from build123d import *

# Parameters (mm, degrees)
BOSS_EXTRUDE1_DEPTH = 15
CUT_EXTRUDE2_DEPTH  = 10
FILLET2_R           = 2


with BuildPart() as part:
    # Sketch1 → Boss-Extrude1 (new body)
    with BuildSketch(Plane(origin=(0, 0, 0), x_dir=(1, 0, 0), z_dir=(0, 1, 0))):
        Polygon((-2, 0), (-2, 30), (-11, 30), (-11, 35), (2, 35), (2, 30), (2, 0), (-4.698729811, -25), (-8.698729811, -25), (-3.876557728, -7.003408785), (-18.977490779, -25), (-22.977490779, -25), align=None)
    extrude(amount=BOSS_EXTRUDE1_DEPTH)

    # Sketch3 → Cut-Extrude2 (cut)
    with BuildSketch(Plane(origin=(0, 0, -35), x_dir=(-1, 0, 0), z_dir=(0, 0, -1))):
        with BuildLine():
            ThreePointArc((8.85, 7.5), (8.611041293, 8.341169779), (7.965541753, 8.931083506))
            Line((7.965541753, 8.931083506), (6.534458247, 6.068916494))
            ThreePointArc((6.534458247, 6.068916494), (8.091169779, 6.138958707), (8.85, 7.5))
        make_face()
        with BuildLine():
            Line((6.534458247, 6.068916494), (7.965541753, 8.931083506))
            ThreePointArc((7.965541753, 8.931083506), (5.818916494, 8.215541753), (6.534458247, 6.068916494))
        make_face()
    extrude(amount=-CUT_EXTRUDE2_DEPTH, mode=Mode.SUBTRACT)

    # Fillet2
    fillet2_edges = [part.edges().sort_by_distance(p)[0] for p in [
        (-2, 7.5, 0),
        (-2, 7.5, -30),
        (2, 7.5, 0),
        (-3.876557728, 7.5, 7.003408785),
    ]]
    fillet(fillet2_edges, radius=FILLET2_R)


solid = part.part
For this review, take the finished solid that the model builds, in its own axes (mm). A direction names the side the tool comes from. Round coordinates to 2 decimals unless told otherwise and drop trailing zeros. Loops run counter-clockwise (first coordinate to the right, second up) from the corner with the lowest first, then second, coordinate; pieces in that order, holes last. Notation, with made-up numbers: (-11.75, 25) - (34.25, 25) arc R26 ccw to (34.25, 62) - close; hole circle Ø9 at (6.25, -27). An arc over 180 degrees is marked (long way). Use one line per item in the form item = value.
1) We need section A-A on x = -7.25. Write out the cut boundary in (y, z).
Solutions:
outline = (0, -35) - (5.9, -35) - (5.9, -30) - (0, -30) - close; (0, 6.26) - (15, 6.26) - (15, 13.41) - (0, 13.41) - close; (0, 19.59) - (15, 19.59) - (15, 25) - (0, 25) - close; (9.1, -35) - (15, -35) - (15, -30) - (9.1, -30) - close
2) Tool access review of faces 5 (the face through (-14.26, 7.4, 19.38)), 6 (the face through (-7.47, 7.4, 20.42)), 7 (the face through (-1, 15, -3)), 8 (the face through (-9, 7, -30)): name each direction out of +Z, -Z, +X, -X, +Y, -Y from which nothing blocks a thin tool from reaching the whole face with its end or side.
Solutions:
face_5 = +Z, +Y, -Y
face_6 = +Y, -Y
face_7 = +Z, -Z, +X, -X, +Y
face_8 = -X, +Y, -Y
3) We need section D-D on z = -5.5. Write out the cut boundary in (x, y).
Solutions:
outline = (-2, 0) - (2, 0) - (2, 15) - (-2, 15) - close
4) Clearance check with flat-ended pins moving along their axes: P1, Ø1.5, axis at x = -2.5, z = -26.5, coming from the +Y side; P2, Ø2, axis at y = 11.5, z = 1.5, coming from the -X side; P3, Ø4, axis at y = 10, z = -31.5, coming from the -X side. State where each tip first meets the part, or that it passes through.
Solutions:
P1 = 15
P2 = -4.1
P3 = -11
5) Wall thickness on probe 1 along X at (y, z) = (11, -20); probe 2 along Z at (x, y) = (-9.75, 3.5); probe 3 along X at (y, z) = (9.75, 23): over which ranges is each line inside the solid? List them lowest first.
Solutions:
probe_1 = -2 to 2
probe_2 = -35 to -30, 9.24 to 14
probe_3 = -21.3 to -17.3, -8.16 to -4.16
6) We need section B-B on y = 14. Write out the cut boundary in (x, z).
Solutions:
outline = (-22.98, 25) - (-2.47, 0.56) arc R2 cw to (-2, -0.73) - (-2, -28) arc R2 cw to (-4, -30) - (-11, -30) - (-11, -35) - (2, -35) - (2, -0.26) arc R2 ccw to (1.93, 0.25) - (-4.7, 25) - (-8.7, 25) - (-6.21, 15.72) arc R2 cw to (-9.68, 13.91) - (-18.98, 25) - close
7) Mouldability with a two-part tool opening along Z and no side actions: class faces 1 (the face through (-2.57, 7.6, -29.4)), 2 (the face through (-11, 7, -32)), 3 (the face through (-5, 7, -35)), 4 (the face through (-1.337, 7.395, 12.454)) as pulls with the +Z half, pulls with the -Z half, needs draft (parallel to the pull), parting line crosses it, or undercut.
Solutions:
face_1 = undercut
face_2 = needs draft
face_3 = pulls with the -Z half
face_4 = pulls with the +Z half
8) We need section C-C on z = 19. Write out the cut boundary in (x, y), then the cut area to 3 significant figures.
Solutions:
outline = (-17.94, 0) - (-13.94, 0) - (-13.94, 15) - (-17.94, 15) - close; (-7.09, 0) - (-3.09, 0) - (-3.09, 15) - (-7.09, 15) - close
area = 120 mm2
